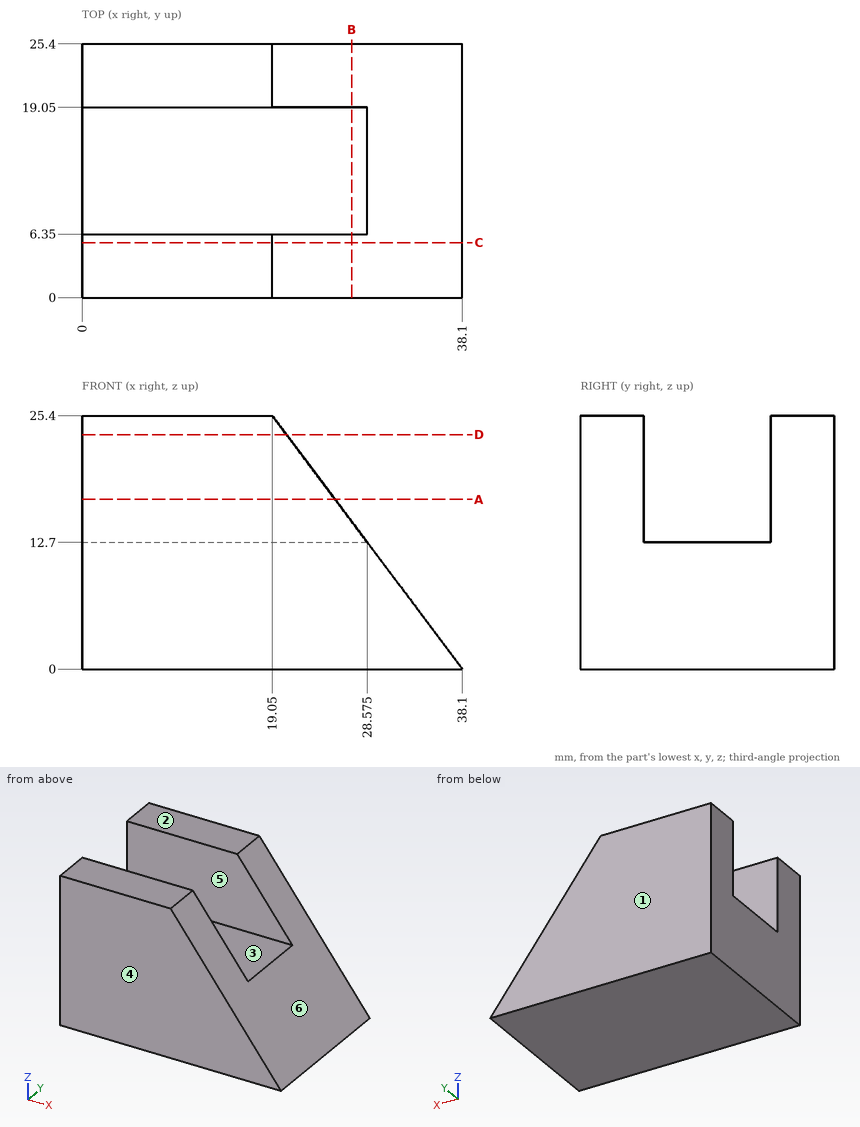
Answer from the drawing. Dimensions are ordinates in mm from the lowest x, y and z of the part. A direction names the side the tool comes from. Round coordinates to 2 decimals unless told otherwise and drop trailing zeros. Loops run counter-clockwise (first coordinate to the right, second up) from the corner with the lowest first, then second, coordinate; pieces in that order, holes last. Notation, with made-up numbers: M -9.5,-16.75 L 3.5,-16.75 A11 ccw 3.5,-10.75 Z; hole C 17.25,54.25 d9. An arc over 180 degrees is marked long. One line per question, with ' | ' between items. Start each with the question number.
(1) For a pull along Y with two mould halves and no side action, classify the marked faces 1, 2, 3 and 4 as released by +Y, released by -Y, zero draft, split by the parting line, or undercut.
(2) A cutting plane is placed at B-B on x = 27. Write down the section's boundary in (y, z), plus the area to 3 significant figures.
(3) A cutting plane is placed at A-A on z = 17. Write down the section's boundary in (x, y).
(4) A cutting plane is placed at C-C on y = 5.5. Write down the section's boundary in (x, z).
(5) A tool of negligible diameter and unlimited length cuts with its end or side. For the marked faces 5 and 6, from which of +Z, -Z, +X, -X, +Y, -Y can it reach the whole face along a straight path? Write none if from no direction.
(6) Find the intervals of material crossed by line 1 (Y direction, x = 6, z = 18.25); line 2 (Z direction, x = 4.5, y = 15.5); line 3 (X direction, y = 9.5, z = 4.5) (3 decimals), in increasing order.
(7) A cutting plane is placed at D-D on z = 23.5. Write down the section's boundary in (x, y) (3 decimals), plus the area to 3 significant figures.
Geometry check:
1) face 1: released by +Y | face 2: zero draft | face 3: undercut | face 4: released by -Y
2) outline: M 0,0 L 25.4,0 L 25.4,14.8 L 19.05,14.8 L 19.05,12.7 L 6.35,12.7 L 6.35,14.8 L 0,14.8 Z | area: 349 mm²
3) outline: M 0,0 L 25.35,0 L 25.35,6.35 L 0,6.35 Z; M 0,19.05 L 25.35,19.05 L 25.35,25.4 L 0,25.4 Z
4) outline: M 0,0 L 38.1,0 L 19.05,25.4 L 0,25.4 Z
5) face 5: +Z, +X, -X | face 6: +Z, +X, +Y, -Y
6) line 1: y = 0 to 6.35, 19.05 to 25.4 | line 2: z = 0 to 12.7 | line 3: x = 0 to 34.725
7) outline: M 0,0 L 20.475,0 L 20.475,6.35 L 0,6.35 Z; M 0,19.05 L 20.475,19.05 L 20.475,25.4 L 0,25.4 Z | area: 260 mm²
